Print and shaded views of the part. All mm, measured from the part's lowest x, y and z. A direction names the side the tool comes from. Give positions to 0.01 mm unless a question says otherwise; leave off trailing zeros. Loops run counter-clockwise (first coordinate to the right, second up) from the corner with the lowest first, then second, coordinate; pieces in that order, holes last. Notation, with made-up numbers: M 26,-28.5 L 33,-28.5 A23 ccw 33,4.5 Z; hole C 86,84.25 d6. An arc over 180 degrees is marked long. Put each result on its own line as item: value. Start each with the question number.
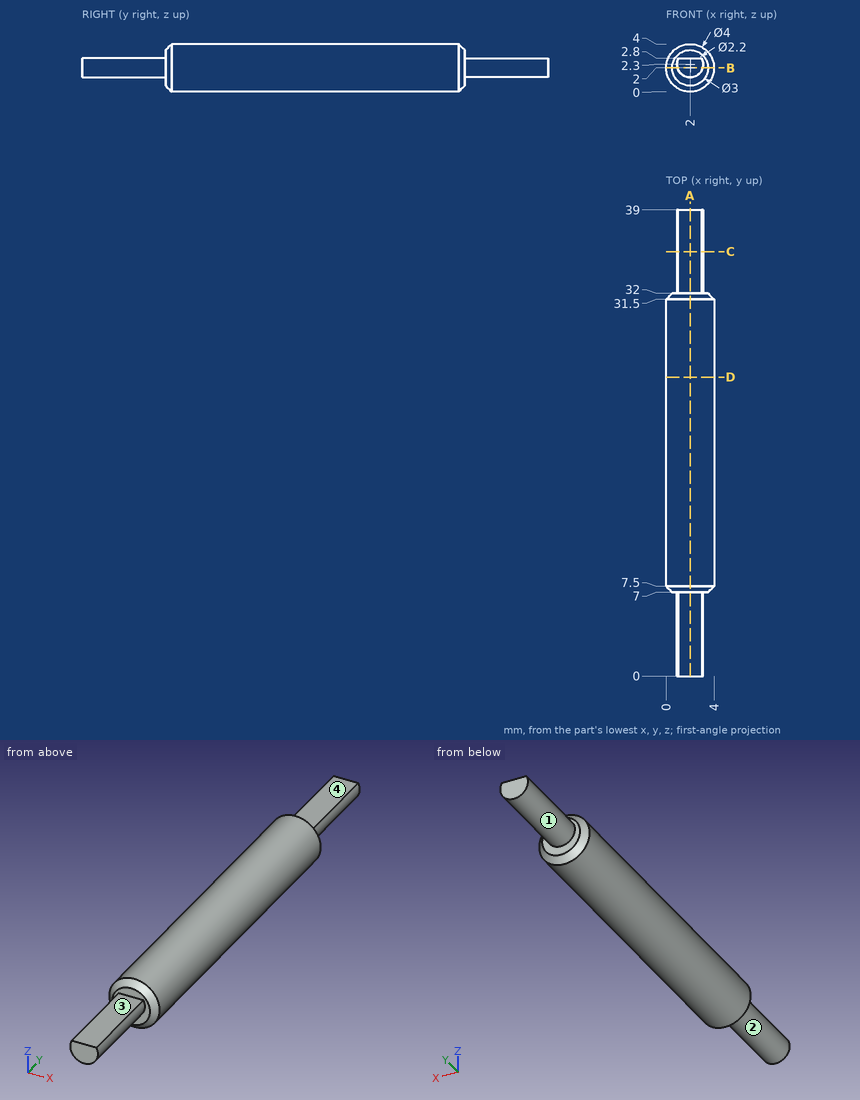
1) Pin check, flat tips, straight feed: pin 1 Ø0.6 at (x, y) = (2, 34.5) entering from +Z; pin 2 Ø1.5 at (x, z) = (2, 1.5) entering from -Y. Stop position of each tip, or through.
2) Band-saw the part on A-A on x = 2. Give the cut face in (y, z), then the cut area to 3 significant figures.
3) Band-saw the part on C-C on y = 35.5. Give the cut face in (x, z).
4) Wall check: L1, parallel to Y at x = 1.6, z = 1.1; L2, parallel to X at y = 33.5, z = 2.2; L3, parallel to Z at x = 2.45, y = 23. Give the ranges that are in metal, low to high.
5) Band-saw the part on B-B on z = 2. Give the cut face in (x, y).
6) Which spindle directions (+Z, -Z, +X, -X, +Y, -Y) get a long thin tool onto all of the face, cutting with end or side? Do the marked faces 1, 2, 3 and 4. Say none if no direction does.
7) Band-saw the part on D-D on y = 25. Give the cut face in (x, z), then the cut area to 3 significant figures.
Evaluation:
1. pin 1: z = 2.8
1. pin 2: y = 0
2. outline: M 0,1.2 L 7,1.2 L 7,0.5 L 7.5,0 L 31.5,0 L 32,0.5 L 32,1.2 L 39,1.2 L 39,2.8 L 32,2.8 L 32,3.5 L 31.5,4 L 7.5,4 L 7,3.5 L 7,2.8 L 0,2.8 Z
2. area: 122 mm2
3. outline: M 1.02,2.8 A1.1 ccw long 2.98,2.8 Z
4. L1: 7 to 32
4. L2: 0.9 to 3.1
4. L3: 0.05 to 3.95
5. outline: M 0,7.5 L 0.5,7 L 0.94,7 L 0.94,0 L 3.06,0 L 3.06,7 L 3.5,7 L 4,7.5 L 4,31.5 L 3.5,32 L 3.06,32 L 3.06,39 L 0.94,39 L 0.94,32 L 0.5,32 L 0,31.5 Z
6. face 1: +Y
6. face 2: -Y
6. face 3: +Z, +X, -X, -Y
6. face 4: +Z, +X, -X, +Y
7. outline: C 2,2 d4
7. area: 12.6 mm2
